```python
from build123d import *

# Parameters (mm, degrees)
SKETCH1_W           = 200
SKETCH1_H           = 125
BOSS_EXTRUDE3_DEPTH = 40
BOSS_EXTRUDE4_DEPTH = 10
EXTRUDE_THIN1_DEPTH = 40
SKETCH5_W           = 30
SKETCH5_H           = 15
CUT_EXTRUDE2_DEPTH  = 40
SKETCH6_W           = 210
SKETCH6_H           = 135
CUT_EXTRUDE3_DEPTH  = 20
SKETCH7_R           = 10
BOSS_EXTRUDE5_DEPTH = 5
SKETCH8_R           = 1.7
CUT_EXTRUDE5_DEPTH  = 5
SKETCH9_W           = 10
SKETCH9_H           = 5
CUT_EXTRUDE6_DEPTH  = 10
SKETCH10_W          = 230
SKETCH10_H          = 155
BOSS_EXTRUDE6_DEPTH = 10
SKETCH12_W          = 70
SKETCH12_H          = 10
CUT_EXTRUDE7_DEPTH  = 250


with BuildPart() as part:
    # Sketch1 → Boss-Extrude3 (new body)
    with BuildSketch(Plane(origin=(0, 0, 0), x_dir=(1, 0, 0), z_dir=(0, 1, 0))):
        Polygon((5, 0), (0, 0), (0, -135), (210, -135), (210, 0), align=None)
        with Locations((105, -67.5)):
            Rectangle(SKETCH1_W, SKETCH1_H, mode=Mode.SUBTRACT)
    extrude(amount=BOSS_EXTRUDE3_DEPTH)

    # Sketch3 → Boss-Extrude4 (add)
    with BuildSketch(Plane(origin=(0, 0, 0), x_dir=(-1, 0, 0), z_dir=(0, -1, 0))):
        Polygon((-220, -145), (0, -145), (10, -145), (10, 10), (-220, 10), align=None)
    extrude(amount=BOSS_EXTRUDE4_DEPTH)

    # Sketch4 → Extrude-Thin1 (add)
    with BuildSketch(Plane(origin=(0, 0, 0), x_dir=(1, 0, 0), z_dir=(0, 1, 0))):
        Polygon((205, -32.5), (65, -32.5), (65, -102.5), (205, -102.5), (205, -112.5), (55, -112.5), (55, -22.5), (205, -22.5), align=None)
    extrude(amount=EXTRUDE_THIN1_DEPTH)

    # Sketch5 → Cut-Extrude2 (cut)
    with BuildSketch(Plane.ZY.offset(-55)):
        with Locations((82.5, 7.5)):
            Rectangle(SKETCH5_W, SKETCH5_H)
        with Locations((52.5, 7.5)):
            Rectangle(SKETCH5_W, SKETCH5_H)
    extrude(amount=-CUT_EXTRUDE2_DEPTH, mode=Mode.SUBTRACT)

    # Sketch6 → Cut-Extrude3 (cut)
    with BuildSketch(Plane(origin=(0, 40, 0), x_dir=(1, 0, 0), z_dir=(0, 1, 0))):
        with Locations((105, -67.5)):
            Rectangle(SKETCH6_W, SKETCH6_H)
    extrude(amount=-CUT_EXTRUDE3_DEPTH, mode=Mode.SUBTRACT)

    # Sketch7 → Boss-Extrude5 (add)
    with BuildSketch(Plane(origin=(0, 20, 0), x_dir=(1, 0, 0), z_dir=(0, 1, 0))):
        Circle(SKETCH7_R)
        with Locations((210, 0)):
            Circle(SKETCH7_R)
        with Locations((210, -135)):
            Circle(SKETCH7_R)
        with Locations((0, -135)):
            Circle(SKETCH7_R)
    extrude(amount=-BOSS_EXTRUDE5_DEPTH)

    # Sketch8 → Cut-Extrude5 (cut)
    with BuildSketch(Plane(origin=(0, 20, 0), x_dir=(1, 0, 0), z_dir=(0, 1, 0))):
        with Locations(Location((-3.535533906, 3.535533906, 0), (0, 0, 270))):
            Circle(SKETCH8_R)
        with Locations(Location((213.535533906, 3.535533906, 0), (0, 0, 270))):
            Circle(SKETCH8_R)
        with Locations(Location((213.535533906, -138.535533906, 0), (0, 0, 270))):
            Circle(SKETCH8_R)
        with Locations(Location((-3.535533906, -138.535533906, 0), (0, 0, 270))):
            Circle(SKETCH8_R)
    extrude(amount=-CUT_EXTRUDE5_DEPTH, mode=Mode.SUBTRACT)

    # Sketch9 → Cut-Extrude6 (cut)
    with BuildSketch(Plane.ZY):
        Polygon((77.5, 15.5), (77.5, 10.5), (67.5, 10.5), (57.5, 10.5), (57.5, 15.5), align=None)
        with Locations((72.5, 8)):
            Rectangle(SKETCH9_W, SKETCH9_H)
        with Locations((62.5, 8)):
            Rectangle(SKETCH9_W, SKETCH9_H)
    extrude(amount=-CUT_EXTRUDE6_DEPTH, mode=Mode.SUBTRACT)

    # Sketch10 → Boss-Extrude6 (add)
    with BuildSketch(Plane(origin=(0, 0, 0), x_dir=(1, 0, 0), z_dir=(0, 1, 0))):
        Polygon((230, 20), (-10, 20), (-20, 20), (-20, -225), (230, -225), align=None)
        with Locations((105, -67.5)):
            Rectangle(SKETCH10_W, SKETCH10_H, mode=Mode.SUBTRACT)
    extrude(amount=-BOSS_EXTRUDE6_DEPTH)

    # Sketch12 → Cut-Extrude7 (cut)
    with BuildSketch(Plane.ZY.offset(20)):
        with Locations((190, -5)):
            Rectangle(SKETCH12_W, SKETCH12_H)
    extrude(amount=-CUT_EXTRUDE7_DEPTH, mode=Mode.SUBTRACT)


solid = part.part
```
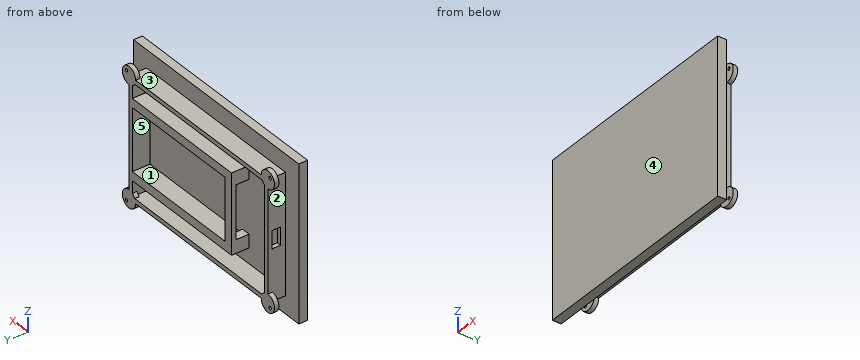
Verification items for the finished model (mm, model axes). Face numbers are marked on the shaded views. A direction names the side the tool comes from. Coordinates: 2 decimals unless noted, no trailing zeros. Loops run counter-clockwise (first coordinate to the right, second up) from the corner with the lowest first, then second, coordinate; pieces in that order, holes last. Notation, with made-up numbers: (-38, 15) - (13, 15) arc R28 cw to (13, 41) - close; hole circle Ø1 at (61, 63). An arc over 180 degrees is marked (long way). Put each result on its own line as item: value.
Item 1: Set-up check for the marked faces 1 and 2: record each of +Z, -Z, +X, -X, +Y, -Y from which the full face is reachable in a straight line by a thin tool's end or side.
Conclusion:
face 1: +Y
face 2: -X
Item 2: Draft check along Z on the marked faces 3, 4 and 5. Enter one of: pulls with the +Z half, pulls with the -Z half, needs draft (parallel to the pull), parting line crosses it, or undercut.
Conclusion:
face 3: pulls with the +Z half
face 4: needs draft
face 5: undercut
Item 3: Section check C-C (x = 62). Enter the section's corners in (y, z).
Conclusion:
outline: (-10, -20) - (0, -20) - (0, 0) - (20, 0) - (20, 5) - (0, 5) - (0, 22.5) - (20, 22.5) - (20, 112.5) - (0, 112.5) - (0, 130) - (20, 130) - (20, 135) - (0, 135) - (0, 155) - (-10, 155) - close; hole (0, 37.5) - (15, 37.5) - (15, 97.5) - (0, 97.5) - close
Item 4: Section check B-B (z = 74). Enter the section's corners in (x, y), then the cut area to 3 significant figures.
Conclusion:
outline: (-20, -10) - (230, -10) - (230, 0) - (210, 0) - (210, 20) - (205, 20) - (205, 0) - (5, 0) - (5, 5.5) - (0, 5.5) - (0, 0) - (-20, 0) - close; (0, 15.5) - (5, 15.5) - (5, 20) - (0, 20) - close; (55, 15) - (65, 15) - (65, 20) - (55, 20) - close
area: 2,700 mm2
Item 5: Section check A-A (z = 47). Enter the section's corners in (x, y), then the cut area to 3 significant figures.
Conclusion:
outline: (-20, -10) - (230, -10) - (230, 0) - (210, 0) - (210, 20) - (205, 20) - (205, 0) - (5, 0) - (5, 20) - (0, 20) - (0, 0) - (-20, 0) - close; (55, 15) - (65, 15) - (65, 20) - (55, 20) - close
area: 2,750 mm2
Item 6: Gauge pin test, flat ends, axial feed: pin 1 Ø6 at (y, z) = (14, 86.5) entering from -X; pin 2 Ø16 at (y, z) = (14.5, 83) entering from +X; pin 3 Ø10 at (x, y) = (48, 16.5) entering from -Z; pin 4 Ø5.5 at (x, z) = (213.54, -3.54) entering from +Y. Record the tip position at first contact, or that the pin passes through.
Conclusion:
pin 1: stops at x = 0
pin 2: stops at x = 210
pin 3: stops at z = 0
pin 4: stops at y = 20
Item 7: Scan lines: line 1 along Z through (x, y) = (120.5, 2.75); line 2 along X through (y, z) = (17.5, 90.5); line 3 along Z through (x, y) = (20, 6). Record each from-to range of solid material in increasing order.
Conclusion:
line 1: z = 0 to 5, 22.5 to 32.5, 102.5 to 112.5, 130 to 135
line 2: x = 0 to 5, 55 to 65, 205 to 210
line 3: z = 0 to 5, 130 to 135
